from build123d import *

# Parameters (mm, degrees)
ESQUISSE2_W             = 20
ESQUISSE2_H             = 10
BOSS_EXTRU_1_DEPTH      = 10
ENL_V_MAT_EXTRU_2_DEPTH = 10


with BuildPart() as part:
    # Esquisse1 → Révolution3 (revolve)
    with BuildSketch(Plane.XY):
        with BuildLine():
            Line((0, 0), (-20, 0))
            ThreePointArc((-20, 0), (-36.400549446, 42.543014128), (0, 70))
            Line((0, 70), (0, 67))
            ThreePointArc((0, 67), (-33.398032448, 42.122428112), (-19.123657749, 3))
            Line((-19.123657749, 3), (0, 3))
            Line((0, 3), (0, 0))
        make_face()
    revolve(axis=Axis((0, 0, 0), (0, 1, 0)))

    # Esquisse2 → Boss.-Extru.1 (add)
    with BuildSketch(Plane.XZ):
        Rectangle(ESQUISSE2_W, ESQUISSE2_H)
    extrude(amount=BOSS_EXTRU_1_DEPTH)

    # Esquisse3 → Enlèv. mat.-Extru.2 (cut)
    with BuildSketch(Plane(origin=(0, 0, -5), x_dir=(-1, 0, 0), z_dir=(0, 0, -1))):
        Polygon((7, -3), (7, 0), (-7, 0), (-7, -3), (-7, -7), (7, -7), align=None)
    extrude(amount=-ENL_V_MAT_EXTRU_2_DEPTH, mode=Mode.SUBTRACT)


solid = part.part
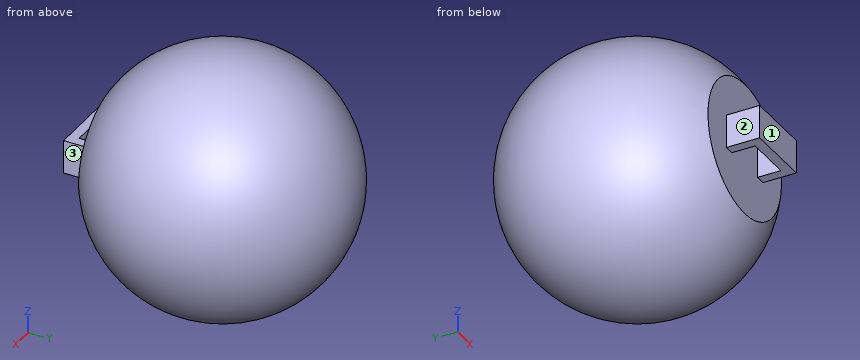
Part model, mm, in its own coordinate system. Face numbers are marked on the shaded views. A direction names the side the tool comes from. Coordinates: 2 decimals unless noted, no trailing zeros. Order: outer loops, then holes, each group sorted by start corner. A loop starts at its lowest first (then second) coordinate and runs counter-clockwise, first axis right, second up.
(1) Tool access for the marked faces 1, 2 and 3: list every direction of +Z, -Z, +X, -X, +Y, -Y with a clear straight run to the whole face (end or side of a thin tool).
Check sheet entries:
face 1: +Z, -Z, +X, -X, -Y
face 2: +Z, -Z, -X, -Y
face 3: +Z, -Z, +X, -Y
(2) Pin check, flat tips, straight feed: pin 1 Ø7.5 at (y, z) = (-4, 2) entering from -X; pin 2 Ø7.5 at (y, z) = (-3, 1) entering from +X; pin 3 Ø1 at (x, z) = (-19.5, 26.5) entering from -Y. Stop position of each tip, or through.
Check sheet entries:
pin 1: stops at x = -10
pin 2: stops at x = 21.14
pin 3: stops at y = 12.56
(3) Slice it at C-C, the plane z = -12. Write the cut outline in (x, y), and give its area (3 significant figures).
Check sheet entries:
outline: (-16, 0) - (16, 0) arc R35.9 ccw (long way) to start; hole (-14.89, 3) - (14.89, 3) arc R32.73 ccw (long way) to start
area: 676 mm2
(4) Slice it at A-A, the plane x = 5. Write the cut outline in (y, z).
Check sheet entries:
outline: (-10, -5) - (-7, -5) - (-7, 5) - (-10, 5) - close; (0, -19.36) arc R37.53 ccw (long way) to (0, 19.36) - close; hole (3, -18.46) arc R34.5 ccw (long way) to (3, 18.46) - close
(5) Slice it at D-D, the plane x = 15.5. Write the cut outline in (y, z).
Check sheet entries:
outline: (0, -12.64) arc R34.54 ccw (long way) to (0, 12.64) - close; hole (3, -11.2) arc R31.22 ccw (long way) to (3, 11.2) - close
(6) Probe L1, parallel to Z at x = -6.5, y = 13.5; L2, parallel to Z at x = 9, y = 47; L3, parallel to X at y = 8, z = 18. List the from-to ranges inside material, lowest first.
Check sheet entries:
L1: z = -32.3 to -28.73, 28.73 to 32.3
L2: z = -33.64 to -30.22, 30.22 to 33.64
L3: x = -22.94 to -17.55, 17.55 to 22.94
(7) Slice it at B-B, the plane y = -1.5. Write the cut outline in (x, z), and give its area (3 significant figures).
Check sheet entries:
outline: (-10, -5) - (-7, -5) - (-7, 5) - (-10, 5) - close; (7, -5) - (10, -5) - (10, 5) - (7, 5) - close
area: 60.0 mm2
